```python
from build123d import *
from build123d.topology import SkipClean

# Parameters (mm, degrees)
MAIN_BASE_DEPTH                 = 60
HOLES_SKETCH_R                  = 4.25
HOLES_SKETCH_R_2                = 1.5
HOLES_SKETCH_R_3                = 9.5
HOLES_DEPTH                     = 30
BOSS_EXTRUDE3_START             = 40
BOSS_EXTRUDE3_DEPTH             = 40
BOSS_EXTRUDE4_REACH             = 84.462
BOSS_EXTRUDE4_DIRECTION_2_REACH = 84.462
CUT_EXTRUDE2_START              = -20
SKETCH4_R                       = 4.25
SKETCH4_R_2                     = 1.5
CUT_EXTRUDE2_DEPTH              = 20
CUT_EXTRUDE3_REACH              = 107.839


with BuildPart() as part:
    # Sketch1 → Main Base (new body)
    with BuildSketch(Plane(origin=(0, 0, 0), x_dir=(0, 0, -1), z_dir=(1, 0, 0))):
        with BuildLine():
            Line((-40, 20), (40, 20))
            Line((40, 20), (40, -10))
            Line((40, -10), (29.69, -10))
            Line((29.69, -10), (29.69, -5.882040462))
            ThreePointArc((29.69, -5.882040462), (24.69, 7.72), (19.69, -5.882040462))
            Line((19.69, -5.882040462), (19.69, -10))
            Line((19.69, -10), (-19.69, -10))
            Line((-19.69, -10), (-19.69, -5.882040462))
            ThreePointArc((-19.69, -5.882040462), (-24.69, 7.72), (-29.69, -5.882040462))
            Line((-29.69, -5.882040462), (-29.69, -10))
            Line((-29.69, -10), (-40, -10))
            Line((-40, -10), (-40, 20))
        make_face()
    extrude(amount=MAIN_BASE_DEPTH)

    # Holes_Sketch → Holes (cut)
    with BuildSketch(Plane(origin=(0, 20, 0), x_dir=(1, 0, 0), z_dir=(0, 1, 0))):
        with Locations(Location((21.25, 0, 0), (0, 0, 270))):
            Circle(HOLES_SKETCH_R)
        with Locations(Location((21.25, -7.5, 0), (0, 0, 270))):
            Circle(HOLES_SKETCH_R_2)
        with Locations(Location((13.75, 0, 0), (0, 0, 270))):
            Circle(HOLES_SKETCH_R_2)
        with Locations(Location((28.75, 0, 0), (0, 0, 270))):
            Circle(HOLES_SKETCH_R_2)
        with Locations(Location((21.25, 7.5, 0), (0, 0, 270))):
            Circle(HOLES_SKETCH_R_2)
        with Locations((51.5, 0)):
            Circle(HOLES_SKETCH_R_3)
    extrude(amount=-HOLES_DEPTH, mode=Mode.SUBTRACT)

    # Sketch3 → Boss-Extrude3 (add)
    with SkipClean():  # the faces are left unmerged after this step: merging them gives an invalid solid
        with BuildSketch(Plane(origin=(0, 20, 0), x_dir=(1, 0, 0), z_dir=(0, 1, 0)).offset(BOSS_EXTRUDE3_START)):
            with BuildLine():
                ThreePointArc((38.839623499, -8.942307692), (48.607661418, -15.227750245), (60, -12.961481397))
                Line((60, -12.961481397), (60, -7.5))
                Line((60, -7.5), (60, -4.242640687))
                ThreePointArc((60, -4.242640687), (51.933558112, -9.490101547), (43.422252789, -5))
                Line((43.422252789, -5), (40.881619709, -5))
                ThreePointArc((40.881619709, -5), (38.66173579, -6.350167236), (38.839623499, -8.942307692))
            make_face()
            with BuildLine():
                ThreePointArc((60, 12.961481397), (57.122608838, 14.444246946), (54, 15.297058541))
                ThreePointArc((54, 15.297058541), (45.508003067, 14.294963195), (38.839623499, 8.942307692))
                ThreePointArc((38.839623499, 8.942307692), (38.66173579, 6.350167236), (40.881619709, 5))
                Line((40.881619709, 5), (43.422252789, 5))
                ThreePointArc((43.422252789, 5), (51.933558112, 9.490101547), (60, 4.242640687))
                Line((60, 4.242640687), (60, 7.5))
                Line((60, 7.5), (60, 12.961481397))
            make_face()
            with BuildLine():
                Line((60, 34), (54, 34))
                Line((54, 34), (54, 15.297058541))
                ThreePointArc((54, 15.297058541), (57.122608838, 14.444246946), (60, 12.961481397))
                Line((60, 12.961481397), (60, 34))
            make_face()
            Polygon((0, 40), (0, 34), (54, 34), (60, 34), (60, 40), align=None)
        extrude(amount=-BOSS_EXTRUDE3_DEPTH)

    # Boss-Extrude4: up to this face of the body (flat: up to its plane)
    boss_extrude4_end = Plane(part.part.faces().sort_by_distance((49.565869061, 60, 10.678132871))[0])
    # Sketch3<6> → Boss-Extrude4 (add, up to the picked face)
    with BuildSketch(Plane(origin=(0, 20, 0), x_dir=(1, 0, 0), z_dir=(0, 1, 0)), mode=Mode.PRIVATE) as boss_extrude4_sk1:
        with BuildLine():
            Line((60, -7.5), (60, -12.961481397))
            ThreePointArc((60, -12.961481397), (62.567738473, -10.8515052), (64.626647497, -8.242640687))
            Line((64.626647497, -8.242640687), (72.626647497, -8.242640687))
            Line((72.626647497, -8.242640687), (72.626647497, -4.242640687))
            Line((72.626647497, -4.242640687), (60, -4.242640687))
            Line((60, -4.242640687), (60, -7.5))
        make_face()
    boss_extrude4_tool1 = split(extrude(boss_extrude4_sk1.sketch, amount=BOSS_EXTRUDE4_REACH, mode=Mode.PRIVATE), bisect_by=boss_extrude4_end, keep=Keep.BOTH, mode=Mode.PRIVATE)
    # Sketch3<6> → Boss-Extrude4 (add, up to the picked face)
    with BuildSketch(Plane(origin=(0, 20, 0), x_dir=(1, 0, 0), z_dir=(0, 1, 0)), mode=Mode.PRIVATE) as boss_extrude4_sk2:
        with BuildLine():
            ThreePointArc((64.626647497, 8.242640687), (62.567738473, 10.8515052), (60, 12.961481397))
            Line((60, 12.961481397), (60, 7.5))
            Line((60, 7.5), (60, 4.242640687))
            Line((60, 4.242640687), (72.626647497, 4.242640687))
            Line((72.626647497, 4.242640687), (72.626647497, 8.242640687))
            Line((72.626647497, 8.242640687), (64.626647497, 8.242640687))
        make_face()
    boss_extrude4_tool2 = split(extrude(boss_extrude4_sk2.sketch, amount=BOSS_EXTRUDE4_REACH, mode=Mode.PRIVATE), bisect_by=boss_extrude4_end, keep=Keep.BOTH, mode=Mode.PRIVATE)
    add(boss_extrude4_tool1.solids().sort_by(Axis((65.389209, 20, 6.97315), (0, 1, 0)))[0])
    add(boss_extrude4_tool2.solids().sort_by(Axis((65.389209, 20, -6.97315), (0, 1, 0)))[0])

    # Boss-Extrude4 direction 2: up to this face of the body (flat: up to its plane)
    boss_extrude4_direction_2_end = Plane(part.part.faces().sort_by_distance((0.717689654, -10, 0))[0])
    # Sketch3<6> → Boss-Extrude4 direction 2 (add, up to the picked face)
    with BuildSketch(Plane(origin=(0, 20, 0), x_dir=(1, 0, 0), z_dir=(0, 1, 0)), mode=Mode.PRIVATE) as boss_extrude4_direction_2_sk1:
        with BuildLine():
            Line((60, -7.5), (60, -12.961481397))
            ThreePointArc((60, -12.961481397), (62.567738473, -10.8515052), (64.626647497, -8.242640687))
            Line((64.626647497, -8.242640687), (72.626647497, -8.242640687))
            Line((72.626647497, -8.242640687), (72.626647497, -4.242640687))
            Line((72.626647497, -4.242640687), (60, -4.242640687))
            Line((60, -4.242640687), (60, -7.5))
        make_face()
    boss_extrude4_direction_2_tool1 = split(extrude(boss_extrude4_direction_2_sk1.sketch, amount=-BOSS_EXTRUDE4_DIRECTION_2_REACH, mode=Mode.PRIVATE), bisect_by=boss_extrude4_direction_2_end, keep=Keep.BOTH, mode=Mode.PRIVATE)
    # Sketch3<6> → Boss-Extrude4 direction 2 (add, up to the picked face)
    with BuildSketch(Plane(origin=(0, 20, 0), x_dir=(1, 0, 0), z_dir=(0, 1, 0)), mode=Mode.PRIVATE) as boss_extrude4_direction_2_sk2:
        with BuildLine():
            ThreePointArc((64.626647497, 8.242640687), (62.567738473, 10.8515052), (60, 12.961481397))
            Line((60, 12.961481397), (60, 7.5))
            Line((60, 7.5), (60, 4.242640687))
            Line((60, 4.242640687), (72.626647497, 4.242640687))
            Line((72.626647497, 4.242640687), (72.626647497, 8.242640687))
            Line((72.626647497, 8.242640687), (64.626647497, 8.242640687))
        make_face()
    boss_extrude4_direction_2_tool2 = split(extrude(boss_extrude4_direction_2_sk2.sketch, amount=-BOSS_EXTRUDE4_DIRECTION_2_REACH, mode=Mode.PRIVATE), bisect_by=boss_extrude4_direction_2_end, keep=Keep.BOTH, mode=Mode.PRIVATE)
    add(boss_extrude4_direction_2_tool1.solids().sort_by(Axis((65.389209, 20, 6.97315), (0, -1, 0)))[0])
    add(boss_extrude4_direction_2_tool2.solids().sort_by(Axis((65.389209, 20, -6.97315), (0, -1, 0)))[0])

    # Sketch4 → Cut-Extrude2 (cut)
    # profile 1 of 5: a face of its own
    with SkipClean():  # the faces are left unmerged after this step: merging them gives an invalid solid
        with BuildSketch(Plane.XZ.offset(10).offset(CUT_EXTRUDE2_START)):
            with Locations(Location((21.25, 0, 0), (0, 0, 90))):
                Circle(SKETCH4_R)
        # profile 2 of 5: a face of its own
        with BuildSketch(Plane.XZ.offset(10).offset(CUT_EXTRUDE2_START)):
            Polygon((31.65, 1.674315781), (28.75, 3.348631561), (25.85, 1.674315781), (25.85, -1.674315781), (28.75, -3.348631561), (31.65, -1.674315781), align=None)
            with Locations(Location((28.75, 0, 0), (0, 0, 90))):
                Circle(SKETCH4_R_2, mode=Mode.SUBTRACT)
        # profile 3 of 5: a face of its own
        with BuildSketch(Plane.XZ.offset(10).offset(CUT_EXTRUDE2_START)):
            Polygon((22.924315781, 4.6), (24.598631561, 7.5), (22.924315781, 10.4), (19.575684219, 10.4), (17.901368439, 7.5), (19.575684219, 4.6), align=None)
            with Locations(Location((21.25, 7.5, 0), (0, 0, 90))):
                Circle(SKETCH4_R_2, mode=Mode.SUBTRACT)
        # profile 4 of 5: a face of its own
        with BuildSketch(Plane.XZ.offset(10).offset(CUT_EXTRUDE2_START)):
            Polygon((22.924315781, -10.4), (24.598631561, -7.5), (22.924315781, -4.6), (19.575684219, -4.6), (17.901368439, -7.5), (19.575684219, -10.4), align=None)
            with Locations(Location((21.25, -7.5, 0), (0, 0, 90))):
                Circle(SKETCH4_R_2, mode=Mode.SUBTRACT)
        # profile 5 of 5: a face of its own
        with BuildSketch(Plane.XZ.offset(10).offset(CUT_EXTRUDE2_START)):
            Polygon((10.85, -1.674315781), (13.75, -3.348631561), (16.65, -1.674315781), (16.65, 1.674315781), (13.75, 3.348631561), (10.85, 1.674315781), align=None)
            with Locations(Location((13.75, 0, 0), (0, 0, 90))):
                Circle(SKETCH4_R_2, mode=Mode.SUBTRACT)
        extrude(amount=CUT_EXTRUDE2_DEPTH, mode=Mode.SUBTRACT)

    # Cut-Extrude3: up to this face of the body (flat: up to its plane)
    cut_extrude3_end = Plane(part.part.faces().sort_by_distance((68.626647497, 40, 8.242640687))[0])
    # Sketch7 → Cut-Extrude3 (cut, up to the picked face)
    with BuildSketch(Plane(origin=(0, 0, -8.242640687), x_dir=(-1, 0, 0), z_dir=(0, 0, -1)), mode=Mode.PRIVATE) as cut_extrude3_sk1:
        with BuildLine():
            Line((-66.876647497, 50), (-66.876647497, 42))
            ThreePointArc((-66.876647497, 42), (-68.626647497, 40.25), (-70.376647497, 42))
            Line((-70.376647497, 42), (-70.376647497, 50))
            ThreePointArc((-70.376647497, 50), (-68.626647497, 51.75), (-66.876647497, 50))
        make_face()
    cut_extrude3_tool1 = split(extrude(cut_extrude3_sk1.sketch, amount=-CUT_EXTRUDE3_REACH, mode=Mode.PRIVATE), bisect_by=cut_extrude3_end, keep=Keep.BOTH, mode=Mode.PRIVATE)
    # Sketch7 → Cut-Extrude3 (cut, up to the picked face)
    with BuildSketch(Plane(origin=(0, 0, -8.242640687), x_dir=(-1, 0, 0), z_dir=(0, 0, -1)), mode=Mode.PRIVATE) as cut_extrude3_sk2:
        with BuildLine():
            Line((-66.876647497, 30), (-66.876647497, 22))
            ThreePointArc((-66.876647497, 22), (-68.626647497, 20.25), (-70.376647497, 22))
            Line((-70.376647497, 22), (-70.376647497, 30))
            ThreePointArc((-70.376647497, 30), (-68.626647497, 31.75), (-66.876647497, 30))
        make_face()
    cut_extrude3_tool2 = split(extrude(cut_extrude3_sk2.sketch, amount=-CUT_EXTRUDE3_REACH, mode=Mode.PRIVATE), bisect_by=cut_extrude3_end, keep=Keep.BOTH, mode=Mode.PRIVATE)
    # Sketch7 → Cut-Extrude3 (cut, up to the picked face)
    with BuildSketch(Plane(origin=(0, 0, -8.242640687), x_dir=(-1, 0, 0), z_dir=(0, 0, -1)), mode=Mode.PRIVATE) as cut_extrude3_sk3:
        with BuildLine():
            Line((-66.876647497, 10), (-66.876647497, 2))
            ThreePointArc((-66.876647497, 2), (-68.626647497, 0.25), (-70.376647497, 2))
            Line((-70.376647497, 2), (-70.376647497, 10))
            ThreePointArc((-70.376647497, 10), (-68.626647497, 11.75), (-66.876647497, 10))
        make_face()
    cut_extrude3_tool3 = split(extrude(cut_extrude3_sk3.sketch, amount=-CUT_EXTRUDE3_REACH, mode=Mode.PRIVATE), bisect_by=cut_extrude3_end, keep=Keep.BOTH, mode=Mode.PRIVATE)
    add(cut_extrude3_tool1.solids().sort_by(Axis((68.626647, 46, -8.242641), (0, 0, 1)))[0], mode=Mode.SUBTRACT)
    add(cut_extrude3_tool2.solids().sort_by(Axis((68.626647, 26, -8.242641), (0, 0, 1)))[0], mode=Mode.SUBTRACT)
    add(cut_extrude3_tool3.solids().sort_by(Axis((68.626647, 6, -8.242641), (0, 0, 1)))[0], mode=Mode.SUBTRACT)


solid = part.part
```
The model under review builds one solid part; all positions refer to its coordinate system, in mm. A direction names the side the tool comes from. Coordinates: 2 decimals unless noted, no trailing zeros. Order: outer loops, then holes, each group sorted by start corner. A loop starts at its lowest first (then second) coordinate and runs counter-clockwise, first axis right, second up. Notation, with made-up numbers: (71, 34.25) -> (95, 34.25) arc R30 ccw to (95, 64.25) -> close; hole circle Ø6 at (66, -31). An arc over 180 degrees is marked (long way). Answer in a Markdown table with one row per item. Add a question column.
Item 1: We need section B-B on z = -24.69. Write out the cut boundary in (x, y).
Item 2: Clearance check with flat-ended pins moving along their axes: pin 1 (3 mm diameter, centred on y = 26, z = -7, fed in from -X); pin 2 (1 mm diameter, centred on x = 30, z = 14.5, fed in from +Y); pin 3 (4.5 mm diameter, centred on x = 21.5, z = -7, fed in from -Y); pin 4 (14 mm diameter, centred on x = 63.5, y = 22, fed in from -Z). State where each tip first meets the part, or that it passes through.
Item 3: We need section A-A on y = 39. Write out the cut boundary in (x, z).
Item 4: To check wall thickness, follow probe 1 along X at (y, z) = (11.75, 0); probe 2 along X at (y, z) = (1, 0); probe 3 along Z at (x, y) = (66, 51). State the ranges of each line that lie inside material, in increasing order.
Item 5: Mouldability with a two-part tool opening along X and no side actions: class faces 1 (the flat face through (66, 25, 4.243)), 2 (the cylindrical face through (55.061, 33.268, 15.085)), 3 (the flat face through (18.727, 0.14, -8.93)) as +X half, -X half, draft (parallel to the pull), parting line (faces both ways), or undercut.
Item 6: Machinability: for faces 4 (the flat face through (27, 10, -1)), 5 (the flat face through (30, -8, -19.69)), 6 (the cylindrical face through (68.67, 51.75, -6.27)), 7 (the cylindrical face through (38.68, 40.28, 6.316)), 8 (the flat face through (66, 25, -4.243)), which of the approach directions +Z, -Z, +X, -X, +Y, -Y give a long, thin tool a straight path to every point of the face, cutting with its end or side? Answer none if there is none.
Final values:
| question | item | result |
|---|---|---|
| 1 | outline | (0, 7.72) -> (60, 7.72) -> (60, 60) -> (54, 60) -> (54, 20) -> (0, 20) -> close |
| 2 | pin 1 | stops at x = 38.38 |
| 2 | pin 2 | stops at y = 20 |
| 2 | pin 3 | stops at y = 10 |
| 2 | pin 4 | stops at z = -40 |
| 3 | outline | (0, -40) -> (60, -40) -> (60, -12.96) arc R15.5 ccw to (64.63, -8.24) -> (72.63, -8.24) -> (72.63, -4.24) -> (60, -4.24) arc R9.5 cw to (43.42, -5) -> (40.88, -5) arc R2.5 ccw to (38.84, -8.94) arc R15.5 ccw to (54, -15.3) -> (54, -34) -> (0, -34) -> close; (38.84, 8.94) arc R2.5 ccw to (40.88, 5) -> (43.42, 5) arc R9.5 cw to (60, 4.24) -> (72.63, 4.24) -> (72.63, 8.24) -> (64.63, 8.24) arc R15.5 ccw to start |
| 4 | probe 1 | x = 0 to 12.25, 15.25 to 17, 25.5 to 27.25, 30.25 to 42 |
| 4 | probe 2 | x = 0 to 10.85, 16.65 to 17, 25.5 to 25.85, 31.65 to 42 |
| 4 | probe 3 | z = -8.24 to -4.24, 4.24 to 8.24 |
| 5 | face 1 | draft |
| 5 | face 2 | parting line |
| 5 | face 3 | undercut |
| 6 | face 4 | -Y |
| 6 | face 5 | +X, -X, -Y |
| 6 | face 6 | +Z, -Z |
| 6 | face 7 | -X, +Y |
| 6 | face 8 | +X, +Y, -Y |
